Geometry check sheet. Reference: the model listing, model coordinates, mm. Round coordinates to 2 decimals unless told otherwise and drop trailing zeros. Loops run counter-clockwise (first coordinate to the right, second up) from the corner with the lowest first, then second, coordinate; pieces in that order, holes last. Notation, with made-up numbers: (11.5, -19.5) -> (23.5, -19.5) arc R21 cw to (23.5, -0.5) -> close; hole circle Ø1 at (76.25, 42.5). An arc over 180 degrees is marked (long way). Use one line per item in the form item = value.
from build123d import *

# Parameters (mm, degrees)
F0_R     = 0.374
F1_DEPTH = 1


with BuildPart() as f1:
    # F0 (on Front) → F1 (new body)
    with BuildSketch(Plane.XZ):
        Polygon((-5, -5), (-5, -100.3335), (5, -100.3335), (5, -5), (100.3335, -5), (100.3335, 5), (5, 5), (5, 100.3335), (-5, 100.3335), (-5, 5), (-100.3335, 5), (-100.3335, -5), align=None)
        with Locations((-4.514, -69.5465)):
            Circle(F0_R, mode=Mode.SUBTRACT)
        with Locations((-69.5465, -4.514)):
            Circle(F0_R, mode=Mode.SUBTRACT)
        with Locations((4.514, -69.5465)):
            Circle(F0_R, mode=Mode.SUBTRACT)
        with Locations((69.5465, -4.514)):
            Circle(F0_R, mode=Mode.SUBTRACT)
        with Locations((-69.5465, 4.514)):
            Circle(F0_R, mode=Mode.SUBTRACT)
        with Locations((-4.514, 70.2945)):
            Circle(F0_R, mode=Mode.SUBTRACT)
        with Locations((69.5465, 4.514)):
            Circle(F0_R, mode=Mode.SUBTRACT)
        with Locations((4.514, 70.2945)):
            Circle(F0_R, mode=Mode.SUBTRACT)
    extrude(amount=F1_DEPTH)


solid = f1.part
1. Material ranges on line 1 along X through (y, z) = (-0.3, -17), recorded low to high.
Return value:
line_1 = -5 to 5
2. Section check A-A (z = 55). Record the boundary of the cut face in (x, y).
Return value:
outline = (-5, -1) -> (5, -1) -> (5, 0) -> (-5, 0) -> close
3. Section check B-B (y = -0.8). Count the separate pieces of the cut face and the enclosed holes in it, then the cut area to 3 significant figures.
Return value:
separate_pieces = 1
enclosed_holes = 8
area = 3,910 mm2
4. Section check C-C (x = 37). Record the boundary of the cut face in (y, z), then the cut area to 3 significant figures.
Return value:
outline = (-1, -5) -> (0, -5) -> (0, 5) -> (-1, 5) -> close
area = 10.0 mm2
